Verification items for the finished model (mm, model axes). Face numbers are marked on the shaded views. Round coordinates to 2 decimals unless told otherwise and drop trailing zeros. Write each loop counter-clockwise with the first axis right and the second up, starting at its lowest first coordinate (ties: lowest second). Pieces come first, ordered by that corner, then holes. Notation, with made-up numbers: (-35.5, 26.25) - (19.5, 26.25) arc R14 ccw to (19.5, 30.25) - close; hole circle Ø2 at (-38, 82). An arc over 180 degrees is marked (long way). Answer as a JSON object with one key per item and string values.
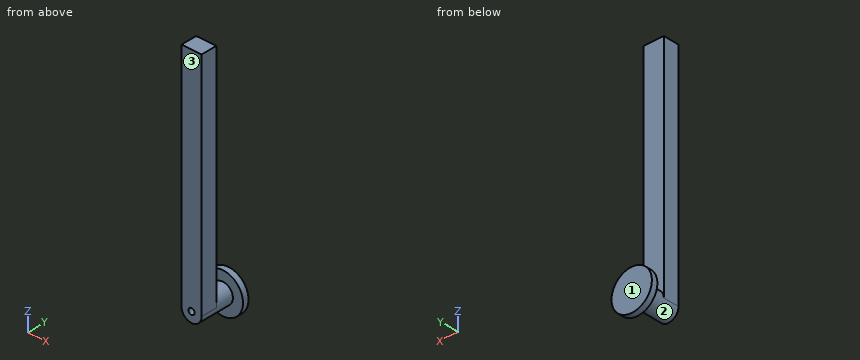
Autodesk Inventor part; units mm, degrees
ref_plane "YZ Plane" through (0, 0, 0) normal (1, 0, 0) x (0, 1, 0)
ref_plane "XZ Plane" through (0, 0, 0) normal (0, 1, 0) x (-1, 0, 0)
ref_plane "XY Plane" through (0, 0, 0) normal (0, 0, 1) x (1, 0, 0)
sketch "Sketch1" plane through (0, 0, 0) normal (0, 1, 0) x (-1, 0, 0)
  line L0 (0, 0) -> (0, -244.795) construction
  line L1 (-5, 0) -> (-5, -244.795)
  line L2 (5, -244.795) -> (5, 0)
  arc A0 (5, 0) -> (-5, 0) centre (0, 0) ccw
  arc A1 (-5, -244.795) -> (5, -244.795) centre (0, -244.795) ccw
  circle A2 centre (0, 0) radius 1.5
  circle A3 centre (0, -244.795) radius 1.5
  point P0 (0, -122.3975)
  dimension "d0" = 244.795
  dimension "d1" = 10
  dimension "d2" = 3
  dimension "d3" = 3
extrude "Extrusion1" add sketch "Sketch1" along normal blind 8
sketch "Sketch2" plane through (0, 8, 0) normal (0, 1, 0) x (1, 0, 0)
  arc A0 (5, 244.795) -> (-5, 244.795) centre (0, 244.795) ccw
  line L0 (-5, 244.795) -> (-5, 0)
  arc A1 (-5, 0) -> (5, 0) centre (0, 0) ccw
  line L1 (5, 0) -> (5, 244.795)
  circle A2 centre (0, 244.795) radius 1.5
  circle A3 centre (0, 0) radius 1.5
  circle A4 centre (0, 244.795) radius 5
  point P0 (-5, 244.795)
  dimension "d12" = 10
extrude "Extrusion2" add sketch "Sketch2" along normal blind 12 contours A4 A0
sketch "Sketch3" plane through (0, 0, 0) normal (0, -1, 0) x (1, 0, 0)
  arc A0 (-5, -244.795) -> (5, -244.795) centre (0, -244.795) ccw
  line L0 (5, 0) -> (5, -244.795)
  arc A1 (5, 0) -> (-5, 0) centre (0, 0) ccw
  line L1 (-5, -244.795) -> (-5, 0)
  circle A2 centre (0, -244.795) radius 1.5
  circle A3 centre (0, 0) radius 1.5
sketch "Sketch4" plane through (0, 20, -244.795) normal (0, 1, 0) x (1, 0, 0)
  circle A0 centre (0, 0) radius 10
  point P0 (0, -244.795)
  dimension "d15" = 20
extrude "Extrusion3" add sketch "Sketch4" against normal blind 3
sketch "Sketch5" plane through (0, 0, 0) normal (0, -1, 0) x (1, 0, 0)
  line L0 (23.0807, 11.4027) -> (-31.8332, 11.4027)
  line L1 (-31.8332, 11.4027) -> (-31.8332, -131.2308)
  line L2 (-31.8332, -131.2308) -> (23.0807, -131.2308)
  line L3 (23.0807, -131.2308) -> (23.0807, 11.4027)
  line L4 (55.5298, 55.2625) -> (-102.4368, 55.2625)
  line L5 (-102.4368, 55.2625) -> (-102.4368, -369.4288)
  line L6 (-102.4368, -369.4288) -> (55.5298, -369.4288)
  line L7 (55.5298, -369.4288) -> (55.5298, 55.2625)
  point P0 (0, 0)
extrude "Extrusion4" cut sketch "Sketch5" against normal blind 100 contours L3 L2 L1 L0
properties part number "Part_12_p2"
1. Cross-section at D-D (y = 14.75). Record the boundary of the cut face in (x, z) (3 decimals).
Completed:
{"outline": "circle Ø10 at (0, -244.795); hole circle Ø3 at (0, -244.795)"}
2. Cross-section at A-A (y = 4.75). Record the boundary of the cut face in (x, z) (3 decimals).
Completed:
{"outline": "(-5, -244.795) arc R5 ccw to (5, -244.795) - (5, -131.231) - (-5, -131.231) - close; hole circle Ø3 at (0, -244.795)"}
3. Cross-section at B-B (z = -221). Record the boundary of the cut face in (x, y), plus the area to 3 significant figures.
Completed:
{"outline": "(-5, 0) - (5, 0) - (5, 8) - (-5, 8) - close", "area": "80.0 mm^2"}
4. Mould release check, pull along Y, two halves, no side actions. Record for the marked faces 1, 2 and 3: released by +Y, released by -Y, zero draft, split by the parting line, or undercut.
Completed:
{"face 1": "released by +Y", "face 2": "undercut", "face 3": "released by -Y"}
5. Go/stop test with flat-tipped pins: pin 1 (4 mm diameter, centred on x = -4.5, z = -218.5, fed in from +Y); pin 2 (12 mm diameter, centred on y = 2.5, z = -228, fed in from +X); pin 3 (6.5 mm diameter, centred on y = 2, z = -195.5, fed in from -X). Record where each tip stops, or that it passes through.
Completed:
{"pin 1": "stops at y = 8", "pin 2": "stops at x = 5", "pin 3": "stops at x = -5"}
6. Cross-section at C-C (x = -7.5). Record the boundary of the cut face in (y, z), plus the area to 3 significant figures.
Completed:
{"outline": "(17, -251.41) - (20, -251.41) - (20, -238.18) - (17, -238.18) - close", "area": "39.7 mm^2"}
7. Material ranges on probe 1 along Z at (x, y) = (0, 12) (3 decimals); probe 2 along Y at (x, z) = (2, -186); probe 3 along Z at (x, y) = (0, 7) (3 decimals), recorded low to high. Write a range as from..to.
Completed:
{"probe 1": "z = -249.795..-246.295, -243.295..-239.795", "probe 2": "y = 0..8", "probe 3": "z = -249.795..-246.295, -243.295..-131.231"}
